Read the model definition and answer for the solid it produces. Units are mm, in the model's axes. Coordinates: 2 decimals unless noted, no trailing zeros. Write each loop counter-clockwise with the first axis right and the second up, starting at its lowest first coordinate (ties: lowest second). Pieces come first, ordered by that corner, then holes. Notation, with made-up numbers: (80.5, 75.5) - (107.5, 75.5) arc R23 cw to (107.5, 89.5) - close; hole circle Ø3 at (58.5, 12.5). An arc over 180 degrees is marked (long way). Return JSON: item names as keys, results as strings.
Autodesk Fusion 360 part; units mm, degrees
sketch "Sketch1" plane through (0, 0, 0) normal (0, 0, 1) x (1, 0, 0)
  line L0 (0, 0) -> (25.4, 0)
  line L1 (25.4, 0) -> (25.4, 25.4)
  line L2 (25.4, 25.4) -> (0, 25.4)
  line L3 (0, 25.4) -> (0, 0)
  dimension "d1" = 25.4
  dimension "d2" = 25.4
extrude "Extrude1" add sketch "Sketch1" along normal blind 914.4 makes body 1
sketch "Sketch2" plane through (0, 0, 914.4) normal (0, 0, 1) x (1, 0, 0)
  line L0 (0, 25.4) -> (0, 0)
  line L1 (0, 0) -> (25.4, 0)
  line L2 (25.4, 0) -> (25.4, 25.4)
  line L3 (25.4, 25.4) -> (0, 25.4)
  line L4 (0, 0) -> (609.6, 0)
  line L5 (609.6, 0) -> (609.6, 914.4)
  line L6 (609.6, 914.4) -> (0, 914.4)
  line L7 (0, 914.4) -> (0, 0)
  dimension "d5" = 609.6
  dimension "d6" = 914.4
sketch "Sketch3" plane through (0, 0, 914.4) normal (0, 0, 1) x (1, 0, 0)
  line L0 (0, 914.4) -> (25.4, 914.4)
  line L1 (25.4, 914.4) -> (25.4, 889)
  line L2 (25.4, 889) -> (0, 889)
  line L3 (0, 889) -> (0, 914.4)
  line L4 (609.6, 914.4) -> (0, 914.4)
  line L5 (0, 914.4) -> (0, 0)
  line L6 (609.6, 914.4) -> (584.2, 914.4)
  line L7 (584.2, 914.4) -> (584.2, 889)
  line L8 (584.2, 889) -> (609.6, 889)
  line L9 (609.6, 889) -> (609.6, 914.4)
  line L10 (609.6, 0) -> (609.6, 914.4)
  line L11 (609.6, 0) -> (584.2, 0)
  line L12 (584.2, 0) -> (584.2, 25.4)
  line L13 (584.2, 25.4) -> (609.6, 25.4)
  line L14 (609.6, 25.4) -> (609.6, 0)
  line L15 (0, 0) -> (609.6, 0)
  dimension "d7" = 25.4
  dimension "d8" = 25.4
  dimension "d9" = 25.4
  dimension "d10" = 25.4
  dimension "d11" = 25.4
  dimension "d12" = 25.4
extrude "Extrude2" add sketch "Sketch3" against normal blind 914.4 separate body contours L0 L1 L2 L3 L4 L5 | L4 L6 L7 L8 L9 L10 | L10 L11 L12 L13 L14 L15 makes body 2 at (25.4, 905.9333, 304.8) makes body 3 at (609.6, 897.4667, 304.8) makes body 4 at (584.2, 8.4667, 304.8)
sketch "Sketch4" plane through (0, 0, 914.4) normal (0, 0, 1) x (1, 0, 0)
  line L0 (584.2, 889) -> (609.6, 889)
  line L1 (609.6, 889) -> (609.6, 25.4)
  line L2 (609.6, 25.4) -> (584.2, 25.4)
  line L3 (584.2, 25.4) -> (584.2, 889)
  line L4 (0, 914.4) -> (584.2, 914.4)
  line L5 (584.2, 914.4) -> (584.2, 889)
  line L6 (584.2, 889) -> (0, 889)
  line L7 (0, 889) -> (0, 914.4)
  line L8 (0, 914.4) -> (25.4, 914.4)
  line L9 (25.4, 914.4) -> (25.4, 0)
  line L10 (25.4, 0) -> (0, 0)
  line L11 (0, 0) -> (0, 914.4)
  line L12 (0, 0) -> (584.2, 0)
  line L13 (584.2, 0) -> (584.2, 25.4)
  line L14 (584.2, 25.4) -> (0, 25.4)
  line L15 (0, 25.4) -> (0, 0)
  line L16 (0, 0) -> (609.6, 0)
  line L17 (0, 914.4) -> (0, 0)
  line L18 (609.6, 914.4) -> (0, 914.4)
  line L19 (609.6, 0) -> (609.6, 914.4)
  line L20 (609.6, 889) -> (609.6, 914.4)
  line L21 (609.6, 914.4) -> (584.2, 914.4)
  dimension "d15" = 25.4
  dimension "d16" = 25.4
  dimension "d17" = 25.4
  dimension "d18" = 25.4
extrude "Extrude3" add sketch "Sketch4" against normal blind 25.4 separate body contours L0 L1 L2 L3 L19 | L4 L5 L6 L9 L18 | L9 L12 L13 L14 L16 | L6 L9 L11 L14 L17 makes body 5 at (397.9333, 897.4667, 914.4)
ref_plane "WorkPlane1" through (596.9, 901.7, 444.5) normal (0, 0, -1) x (-1, 0, 0)
sketch "Sketch5" plane through (0, 0, 444.5) normal (0, 0, -1) x (-1, 0, 0)
  line L0 (-609.6, 1066.8) -> (0, 1066.8)
  line L1 (0, 1066.8) -> (0, 0)
  line L2 (0, 0) -> (-609.6, 0)
  line L3 (-609.6, 0) -> (-609.6, 1066.8)
  line L4 (-584.2, 889) -> (-25.4, 889)
  line L5 (-584.2, 914.4) -> (-584.2, 889)
  line L6 (-584.2, 914.4) -> (-25.4, 914.4)
  line L7 (-25.4, 914.4) -> (-25.4, 889)
  line L8 (-25.4, 889) -> (0, 889)
  line L9 (0, 889) -> (0, 25.4)
  line L10 (-25.4, 25.4) -> (0, 25.4)
  line L11 (-25.4, 889) -> (-25.4, 25.4)
  line L12 (-584.2, 889) -> (-609.6, 889)
  line L13 (-584.2, 25.4) -> (-584.2, 889)
  line L14 (-609.6, 25.4) -> (-584.2, 25.4)
  line L15 (-609.6, 25.4) -> (-609.6, 889)
  line L16 (-25.4, 0) -> (-584.2, 0)
  line L17 (-584.2, 0) -> (-584.2, 25.4)
  line L18 (-584.2, 25.4) -> (-25.4, 25.4)
  line L19 (-25.4, 25.4) -> (-25.4, 0)
  dimension "d22" = 609.6
  dimension "d23" = 1066.8
extrude "Extrude4" add sketch "Sketch5" along normal blind 25.4 separate body contours L3 L12 L13 L14 L15 | L1 L8 L9 L10 L11 | L4 L5 L6 L7 | L2 L16 L17 L18 L19 makes body 6 at (397.9333, 25.4, 436.0333)
ref_plane "WorkPlane2" through (304.8, 901.7, 1727.2) normal (0, 0, 1) x (1, 0, 0)
sketch "Sketch6" plane through (0, 0, 1727.2) normal (0, 0, 1) x (1, 0, 0)
  line L0 (584.2, 889) -> (25.4, 889)
  line L1 (584.2, 914.4) -> (584.2, 889)
  line L2 (25.4, 914.4) -> (584.2, 914.4)
  line L3 (25.4, 889) -> (25.4, 914.4)
  line L4 (0, 889) -> (25.4, 889)
  line L5 (0, 25.4) -> (0, 889)
  line L6 (25.4, 25.4) -> (0, 25.4)
  line L7 (25.4, 889) -> (25.4, 25.4)
  line L8 (584.2, 889) -> (609.6, 889)
  line L9 (584.2, 25.4) -> (584.2, 889)
  line L10 (609.6, 25.4) -> (584.2, 25.4)
  line L11 (609.6, 889) -> (609.6, 25.4)
  line L12 (584.2, 0) -> (25.4, 0)
  line L13 (584.2, 25.4) -> (584.2, 0)
  line L14 (25.4, 25.4) -> (584.2, 25.4)
  line L15 (25.4, 0) -> (25.4, 25.4)
  line L16 (25.4, 25.4) -> (0, 25.4)
  line L17 (25.4, 0) -> (25.4, 25.4)
  line L18 (0, 0) -> (25.4, 0)
  line L19 (0, 25.4) -> (0, 0)
  line L20 (609.6, 25.4) -> (609.6, 0)
  line L21 (584.2, 25.4) -> (609.6, 25.4)
  line L22 (584.2, 0) -> (584.2, 25.4)
  line L23 (609.6, 0) -> (584.2, 0)
  line L24 (609.6, 914.4) -> (609.6, 889)
  line L25 (584.2, 914.4) -> (609.6, 914.4)
  line L26 (584.2, 889) -> (584.2, 914.4)
  line L27 (609.6, 889) -> (584.2, 889)
  line L28 (0, 889) -> (0, 914.4)
  line L29 (25.4, 889) -> (0, 889)
  line L30 (25.4, 914.4) -> (25.4, 889)
  line L31 (0, 914.4) -> (25.4, 914.4)
extrude "Extrude5" add sketch "Sketch6" against normal blind 812.8 contours L1 L8 L24 L25 L26 L27 | L3 L4 L28 L29 L30 L31 | L10 L13 L20 L21 L22 L23 | L6 L15 L16 L17 L18 L19 bodies 1 6 2 3 4 5
extrude "Extrude6" add sketch "Sketch6" against normal blind 25.4 contours L0 L1 L2 L3 L26 L30 | L8 L9 L10 L11 L21 L27 | L4 L5 L6 L7 L16 L29 | L12 L13 L14 L15 L17 L22 bodies 1
combine "Combine1" operation add target body 1 tool bodies 6
sketch "Sketch7" plane through (0, 0, 0) normal (0, -1, 0) x (1, 0, 0)
  line L0 (25.4, 444.5) -> (25.4, 889)
  line L1 (25.4, 889) -> (584.2, 889)
  line L2 (584.2, 889) -> (584.2, 444.5)
  line L3 (584.2, 444.5) -> (25.4, 444.5)
  line L4 (25.4, 419.1) -> (584.2, 419.1)
  line L5 (584.2, 419.1) -> (584.2, 0)
  line L6 (584.2, 0) -> (609.6, 0)
  line L7 (609.6, 0) -> (609.6, 1727.2)
  line L8 (609.6, 1727.2) -> (584.2, 1727.2)
  line L9 (584.2, 1727.2) -> (0, 1727.2)
  line L10 (0, 1727.2) -> (0, 0)
  line L11 (0, 0) -> (25.4, 0)
  line L12 (25.4, 0) -> (25.4, 419.1)
  line L13 (25.4, 1701.8) -> (584.2, 1701.8)
  line L14 (584.2, 1701.8) -> (584.2, 914.4)
  line L15 (584.2, 914.4) -> (25.4, 914.4)
  line L16 (25.4, 914.4) -> (25.4, 1701.8)
  circle A0 centre (457.2, 901.7) radius 6.35
  circle A1 centre (152.4, 901.7) radius 6.35
  line L17 (152.4, 901.7) -> (457.2, 901.7)
  line L18 (152.4, 901.7) -> (152.4, 685.8)
  line L19 (25.4, 711.2) -> (584.2, 711.2)
  line L20 (584.2, 711.2) -> (584.2, 685.8)
  line L21 (584.2, 685.8) -> (25.4, 685.8)
  line L22 (25.4, 685.8) -> (25.4, 711.2)
  dimension "d31" = 12.7
  dimension "d33" = 12.7
  dimension "d34" = 304.8
  dimension "d35" = 152.4
  dimension "d36" = 12.7
  dimension "d37" = 215.9
  dimension "d38" = 25.4
extrude "Extrude7" add sketch "Sketch7" against normal blind 25.4 contours L0 L18 L19 L21 L22 | L2 L18 L19 L20 L21 bodies 1
extrude "Extrude8" add sketch "Sketch7" along normal blind 25.4 contours A0 | A1 L17 L18 | A1 L17 L18 bodies 1
sketch "Sketch8" plane through (0, 0, 1727.2) normal (0, 0, 1) x (1, 0, 0)
  line L0 (0, 914.4) -> (0, 0)
  line L1 (0, 0) -> (584.2, 0)
  line L2 (584.2, 0) -> (609.6, 0)
  line L3 (609.6, 0) -> (609.6, 25.4)
  line L4 (609.6, 25.4) -> (609.6, 889)
  line L5 (609.6, 889) -> (609.6, 914.4)
  line L6 (609.6, 914.4) -> (0, 914.4)
  line L7 (25.4, 25.4) -> (25.4, 889)
  line L8 (25.4, 889) -> (584.2, 889)
  line L9 (584.2, 889) -> (584.2, 25.4)
  line L10 (584.2, 25.4) -> (25.4, 25.4)
  line L11 (6.35, 908.05) -> (603.25, 908.05)
  line L12 (603.25, 908.05) -> (603.25, 6.35)
  line L13 (603.25, 6.35) -> (6.35, 6.35)
  line L14 (6.35, 6.35) -> (6.35, 908.05)
  dimension "d43" = 6.35
  dimension "d44" = 6.35
  dimension "d45" = 6.35
  dimension "d46" = 6.35
extrude "Extrude9" cut sketch "Sketch8" against normal blind 19.05 contours L11 L12 L13 L14 bodies 1
sketch "Sketch9" plane through (0, 0, 914.4) normal (0, 0, 1) x (1, 0, 0)
  line L0 (25.4, 889) -> (0, 889)
  line L1 (0, 889) -> (0, 25.4)
  line L2 (0, 25.4) -> (25.4, 25.4)
  line L3 (25.4, 25.4) -> (25.4, 889)
  line L4 (6.35, 908.05) -> (603.25, 908.05)
  line L5 (603.25, 908.05) -> (603.25, 6.35)
  line L6 (603.25, 6.35) -> (6.35, 6.35)
  line L7 (6.35, 6.35) -> (6.35, 908.05)
  line L8 (25.4, 914.4) -> (25.4, 889)
  line L9 (25.4, 889) -> (584.2, 889)
  line L10 (584.2, 889) -> (584.2, 914.4)
  line L11 (584.2, 914.4) -> (25.4, 914.4)
  line L12 (584.2, 25.4) -> (609.6, 25.4)
  line L13 (609.6, 25.4) -> (609.6, 889)
  line L14 (609.6, 889) -> (584.2, 889)
  line L15 (584.2, 889) -> (584.2, 25.4)
  line L16 (584.2, 0) -> (584.2, 25.4)
  line L17 (584.2, 25.4) -> (25.4, 25.4)
  line L18 (25.4, 25.4) -> (25.4, 0)
  line L19 (25.4, 0) -> (584.2, 0)
  dimension "d49" = 6.35
  dimension "d50" = 6.35
  dimension "d51" = 6.35
  dimension "d52" = 6.35
extrude "Extrude10" cut sketch "Sketch9" against normal blind 19.05 contours L0 L2 L3 L7 | L3 L9 L15 L17 | L4 L8 L9 L10 | L6 L16 L17 L18 | L5 L12 L14 L15 bodies 1
sketch "Sketch10" plane through (0, 0, 711.2) normal (0, 0, 1) x (1, 0, 0)
  line L0 (25.4, 0) -> (584.2, 0)
  line L1 (584.2, 0) -> (584.2, 25.4)
  line L2 (584.2, 25.4) -> (25.4, 25.4)
  line L3 (25.4, 25.4) -> (25.4, 0)
  line L4 (15.2621, 59.1079) -> (599.5555, 59.1079)
  line L5 (599.5555, 59.1079) -> (599.5555, 6.35)
  line L6 (599.5555, 6.35) -> (15.2621, 6.35)
  line L7 (15.2621, 6.35) -> (15.2621, 59.1079)
  dimension "d55" = 6.35
extrude "Extrude11" cut sketch "Sketch10" against normal blind 19.05 contours L1 L2 L3 L6 bodies 1
sketch "Sketch11" plane through (0, 0, 444.5) normal (0, 0, 1) x (1, 0, 0)
  line L0 (584.2, 25.4) -> (25.4, 25.4)
  line L1 (25.4, 25.4) -> (25.4, 0)
  line L2 (25.4, 0) -> (584.2, 0)
  line L3 (584.2, 0) -> (584.2, 25.4)
  line L4 (25.4, 889) -> (0, 889)
  line L5 (0, 889) -> (0, 25.4)
  line L6 (0, 25.4) -> (25.4, 25.4)
  line L7 (25.4, 25.4) -> (25.4, 889)
  line L8 (584.2, 914.4) -> (25.4, 914.4)
  line L9 (584.2, 889) -> (25.4, 889)
  line L10 (609.6, 25.4) -> (609.6, 889)
  line L11 (584.2, 889) -> (584.2, 25.4)
  line L12 (584.2, 25.4) -> (609.6, 25.4)
  line L13 (609.6, 25.4) -> (609.6, 889)
  line L14 (609.6, 889) -> (584.2, 889)
  line L15 (584.2, 889) -> (584.2, 914.4)
  line L16 (584.2, 914.4) -> (25.4, 914.4)
  line L17 (25.4, 914.4) -> (25.4, 889)
  line L18 (25.4, 889) -> (584.2, 889)
  line L19 (6.35, 908.05) -> (603.25, 908.05)
  line L20 (603.25, 908.05) -> (603.25, 6.35)
  line L21 (603.25, 6.35) -> (6.35, 6.35)
  line L22 (6.35, 6.35) -> (6.35, 908.05)
  dimension "d58" = 6.35
  dimension "d59" = 6.35
  dimension "d60" = 6.35
  dimension "d61" = 6.35
extrude "Extrude12" cut sketch "Sketch11" against normal blind 19.05 contours L0 L1 L3 L21 | L11 L12 L14 L20 | L4 L6 L7 L22 | L9 L15 L17 L18 L19 bodies 1
equation "d21 = ( -35 / 2 ) * 1 in"
equation "d34 = 12.5 in - 0.25 in - 0.25 in"
equation "d43 = ( 1 / 4 ) * 1 in"
equation "d44 = d43"
equation "d45 = d44"
equation "d46 = d44"
equation "d47 = -1 in + d44"
equation "d49 = d44"
equation "d50 = d44"
equation "d51 = d44"
equation "d52 = d44"
equation "d53 = -1 in + d44"
equation "d55 = d44"
equation "d56 = -1 in + d44"
equation "d58 = d44"
equation "d59 = d44"
equation "d60 = d44"
equation "d61 = d44"
equation "d62 = -1 in + d44"
(1) Determine the mould class of faces 1 (the face through (10, 0, 860)), 2 (the face through (0, 19, 860)), 3 (the face through (16, 459, 1708.15)) for opening direction Y: +Y half, -Y half, draft (parallel to the pull), parting line (faces both ways), or undercut.
Answer:
{"face 1": "-Y half", "face 2": "draft", "face 3": "undercut"}
(2) Flat-ended cylindrical pins translate along their axes: P1, Ø20.5, axis at x = 394.5, y = 16, coming from the -Z side; P2, Ø12.5, axis at y = 7.5, z = 753.5, coming from the -X side; P3, Ø15, axis at x = 428.5, z = 1720, coming from the -Y side; P4, Ø15, axis at x = 365, y = 14, coming from the +Z side. Find the tip coordinate at first contact, or state that the pin passes through.
Answer:
{"P1": "z = 419.1", "P2": "x = 0", "P3": "y = 0", "P4": "z = 1708.15"}
(3) A straight line is drawn through the part: line 1 (Y direction, x = 69.5, z = 442.5). Find the intervals that lie inside material, in ascending order. Write a range as from..to.
Answer:
{"line 1": "0..6.35, 908.05..914.4"}
(4) A cutting plane is placed at A-A (z = 1044). Determine the outline of the cut face in (x, y).
Answer:
{"outline": "(0, 0) - (25.4, 0) - (25.4, 25.4) - (0, 25.4) - close; (0, 889) - (25.4, 889) - (25.4, 914.4) - (0, 914.4) - close; (584.2, 0) - (609.6, 0) - (609.6, 25.4) - (584.2, 25.4) - close; (584.2, 889) - (609.6, 889) - (609.6, 914.4) - (584.2, 914.4) - close"}
(5) A cutting plane is placed at B-B (x = 497). State how many separate pieces and enclosed holes the cut face has, and give its area (3 significant figures).
Answer:
{"separate pieces": "7", "enclosed holes": "0", "area": "1,980 mm²"}
